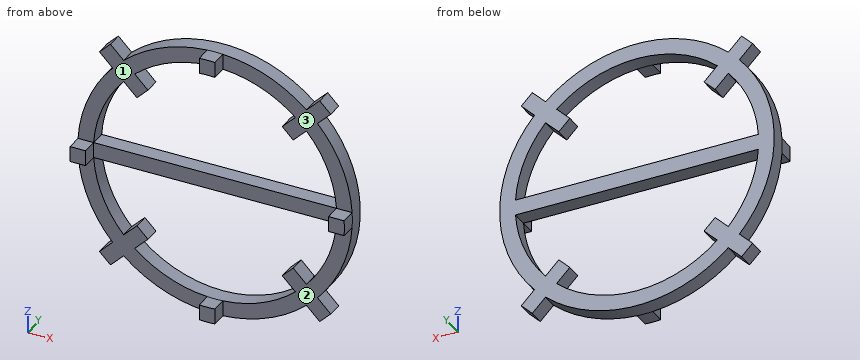
from build123d import *

# Parameters (mm, degrees)
BOSS_EXTRUDE1_DEPTH = 5
BOSS_EXTRUDE2_START = 5
BOSS_EXTRUDE2_DEPTH = 5


with BuildPart() as part:
    # Sketch1 → Boss-Extrude1 (new body)
    with BuildSketch(Plane(origin=(0, 0, 0), x_dir=(1, 0, 0), z_dir=(0, 1, 0))):
        with BuildLine():
            Line((-35.30507781, 35.30507781), (-37.072844763, 33.537310857))
            Line((-37.072844763, 33.537310857), (-32.830204076, 29.29467017))
            ThreePointArc((-32.830204076, 29.29467017), (-44, 0), (-32.830204076, -29.29467017))
            Line((-32.830204076, -29.29467017), (-37.072844763, -33.537310857))
            Line((-37.072844763, -33.537310857), (-35.30507781, -35.30507781))
            Line((-35.30507781, -35.30507781), (-33.537310857, -37.072844763))
            Line((-33.537310857, -37.072844763), (-29.29467017, -32.830204076))
            ThreePointArc((-29.29467017, -32.830204076), (0, -44), (29.29467017, -32.830204076))
            Line((29.29467017, -32.830204076), (33.537310857, -37.072844763))
            Line((33.537310857, -37.072844763), (35.30507781, -35.30507781))
            Line((35.30507781, -35.30507781), (37.072844763, -33.537310857))
            Line((37.072844763, -33.537310857), (32.830204076, -29.29467017))
            ThreePointArc((32.830204076, -29.29467017), (44, 0), (32.830204076, 29.29467017))
            Line((32.830204076, 29.29467017), (37.072844763, 33.537310857))
            Line((37.072844763, 33.537310857), (35.30507781, 35.30507781))
            Line((35.30507781, 35.30507781), (33.537310857, 37.072844763))
            Line((33.537310857, 37.072844763), (29.29467017, 32.830204076))
            ThreePointArc((29.29467017, 32.830204076), (0, 44), (-29.29467017, 32.830204076))
            Line((-29.29467017, 32.830204076), (-33.537310857, 37.072844763))
            Line((-33.537310857, 37.072844763), (-35.30507781, 35.30507781))
        make_face()
        with BuildLine():
            Line((-38.919789311, 2.5), (38.919789311, 2.5))
            ThreePointArc((38.919789311, 2.5), (36.031301768, 14.924653862), (29.288213897, 25.752679991))
            Line((29.288213897, 25.752679991), (25.04557321, 21.510039304))
            Line((25.04557321, 21.510039304), (21.510039304, 25.04557321))
            Line((21.510039304, 25.04557321), (25.752679991, 29.288213897))
            ThreePointArc((25.752679991, 29.288213897), (0, 39), (-25.752679991, 29.288213897))
            Line((-25.752679991, 29.288213897), (-21.510039304, 25.04557321))
            Line((-21.510039304, 25.04557321), (-25.04557321, 21.510039304))
            Line((-25.04557321, 21.510039304), (-29.288213897, 25.752679991))
            ThreePointArc((-29.288213897, 25.752679991), (-36.031301768, 14.924653862), (-38.919789311, 2.5))
        make_face(mode=Mode.SUBTRACT)
        with BuildLine():
            Line((38.919789311, -2.5), (-38.919789311, -2.5))
            ThreePointArc((-38.919789311, -2.5), (-36.031301768, -14.924653862), (-29.288213897, -25.752679991))
            Line((-29.288213897, -25.752679991), (-25.04557321, -21.510039304))
            Line((-25.04557321, -21.510039304), (-21.510039304, -25.04557321))
            Line((-21.510039304, -25.04557321), (-25.752679991, -29.288213897))
            ThreePointArc((-25.752679991, -29.288213897), (0, -39), (25.752679991, -29.288213897))
            Line((25.752679991, -29.288213897), (21.510039304, -25.04557321))
            Line((21.510039304, -25.04557321), (25.04557321, -21.510039304))
            Line((25.04557321, -21.510039304), (29.288213897, -25.752679991))
            ThreePointArc((29.288213897, -25.752679991), (36.031301768, -14.924653862), (38.919789311, -2.5))
        make_face(mode=Mode.SUBTRACT)
    extrude(amount=BOSS_EXTRUDE1_DEPTH)

    # Sketch2 → Boss-Extrude2 (add)
    with BuildSketch(Plane.XZ.offset(BOSS_EXTRUDE2_START)):
        with BuildLine():
            Line((-38.919789311, 2.5), (-43.928919859, 2.5))
            ThreePointArc((-43.928919859, 2.5), (-44, 0), (-43.928919859, -2.5))
            Line((-43.928919859, -2.5), (-38.919789311, -2.5))
            ThreePointArc((-38.919789311, -2.5), (-39, 0), (-38.919789311, 2.5))
        make_face()
        with BuildLine():
            Line((-2.5, 38.919789311), (-2.5, 43.928919859))
            ThreePointArc((-2.5, 43.928919859), (0, 44), (2.5, 43.928919859))
            Line((2.5, 43.928919859), (2.5, 38.919789311))
            ThreePointArc((2.5, 38.919789311), (0, 39), (-2.5, 38.919789311))
        make_face()
        with BuildLine():
            Line((38.919789311, -2.5), (43.928919859, -2.5))
            ThreePointArc((43.928919859, -2.5), (44, 0), (43.928919859, 2.5))
            Line((43.928919859, 2.5), (38.919789311, 2.5))
            ThreePointArc((38.919789311, 2.5), (39, 0), (38.919789311, -2.5))
        make_face()
        with BuildLine():
            Line((2.5, -43.928919859), (2.5, -38.919789311))
            ThreePointArc((2.5, -38.919789311), (0, -39), (-2.5, -38.919789311))
            Line((-2.5, -38.919789311), (-2.5, -43.928919859))
            ThreePointArc((-2.5, -43.928919859), (0, -44), (2.5, -43.928919859))
        make_face()
    extrude(amount=-BOSS_EXTRUDE2_DEPTH)


solid = part.part
Work out the finished part from the listing and answer in its coordinate system (mm). Face numbers are marked on the shaded views. A direction names the side the tool comes from. Round coordinates to 2 decimals unless told otherwise and drop trailing zeros. Order: outer loops, then holes, each group sorted by start corner. A loop starts at its lowest first (then second) coordinate and runs counter-clockwise, first axis right, second up. Notation, with made-up numbers: M -15.75,-26.5 L 27.25,-26.5 A14 cw 27.25,-0.5 Z; hole C -26,-32.75 d2. An arc over 180 degrees is marked long. One line per item, written item: value.
Q1. Find section D-D on x = 35.5. Write down the section's boundary in (y, z).
Derived:
outline: M 0,-35.11 L 5,-35.11 L 5,-31.96 L 0,-31.96 Z; M 0,-26 L 5,-26 L 5,-16.15 L 0,-16.15 Z; M 0,-2.5 L 5,-2.5 L 5,2.5 L 0,2.5 Z; M 0,16.15 L 5,16.15 L 5,26 L 0,26 Z; M 0,31.96 L 5,31.96 L 5,35.11 L 0,35.11 Z
Q2. Flat-ended cylindrical pins translate along their axes: pin 1 (20.5 mm diameter, centred on x = 28.5, z = 24.5, fed in from -Y); pin 2 (1.5 mm diameter, centred on x = 5, y = 3.5, fed in from -Z); pin 3 (1.5 mm diameter, centred on y = -1.5, z = 41, fed in from -X). Find the tip coordinate at first contact, or state that the pin passes through.
Derived:
pin 1: y = 0
pin 2: z = -43.79
pin 3: x = -2.5
Q3. Find section B-B on z = 35. Write down the section's boundary in (x, y).
Derived:
outline: M -35.61,0 L -31.46,0 L -31.46,5 L -35.61,5 Z; M -26.66,0 L -17.2,0 L -17.2,5 L -26.66,5 Z; M 17.2,0 L 26.66,0 L 26.66,5 L 17.2,5 Z; M 31.46,0 L 35.61,0 L 35.61,5 L 31.46,5 Z
Q4. Find section A-A on y = -2.75. Write down the section's boundary in (x, z).
Derived:
outline: M -43.93,-2.5 L -38.92,-2.5 A39 cw -38.92,2.5 L -43.93,2.5 A44 ccw Z; M -2.5,-43.93 A44 ccw 2.5,-43.93 L 2.5,-38.92 A39 cw -2.5,-38.92 Z; M -2.5,38.92 A39 cw 2.5,38.92 L 2.5,43.93 A44 ccw -2.5,43.93 Z; M 38.92,-2.5 L 43.93,-2.5 A44 ccw 43.93,2.5 L 38.92,2.5 A39 cw Z
Q5. Find section C-C on x = 17. Write down the section's boundary in (y, z), then the cut area to 3 significant figures.
Derived:
outline: M 0,-40.58 L 5,-40.58 L 5,-35.1 L 0,-35.1 Z; M 0,-2.5 L 5,-2.5 L 5,2.5 L 0,2.5 Z; M 0,35.1 L 5,35.1 L 5,40.58 L 0,40.58 Z
area: 79.8 mm²
Q6. For the marked faces 1, 2 and 3, determine the directions among +Z, -Z, +X, -X, +Y, -Y from which every point of the face is accessible in a straight line to the end or side of a thin tool.
Derived:
face 1: +Z, -X, -Y
face 2: -Z, +X, -Y
face 3: +Z, +X, -Y
Q7. Straight lines are drawn through the part: line 1 (Z direction, x = -0.5, y = 1.5); line 2 (Z direction, x = -28, y = 2.25); line 3 (Z direction, x = -22, y = 1.75). For each, find the intervals that lie inside material, in ascending order.
Derived:
line 1: -44 to -39, -2.5 to 2.5, 39 to 44
line 2: -33.94 to -24.46, -2.5 to 2.5, 24.46 to 33.94
line 3: -38.11 to -32.2, -25.54 to -24.56, -2.5 to 2.5, 24.56 to 25.54, 32.2 to 38.11
